Design review of the part built by this model. Coordinates are the model's own, in mm. Face numbers are marked on the shaded views. A direction names the side the tool comes from. Give positions to 0.01 mm unless a question says otherwise; leave off trailing zeros. Loops run counter-clockwise (first coordinate to the right, second up) from the corner with the lowest first, then second, coordinate; pieces in that order, holes last. Notation, with made-up numbers: (42.5, -5.5) -> (77.5, -5.5) arc R33 cw to (77.5, 29.5) -> close; hole circle Ø11 at (7, 12). An arc over 180 degrees is marked (long way). Use CSV: the item, a comma, the result in double quotes. Start each with the question number.
Item 1: Wall thickness on line 1 along X through (y, z) = (1.9, 0); line 2 along X through (y, z) = (1.5, 0); line 3 along Y through (x, z) = (-3.5, -0.5): over which ranges is each line inside the solid? List them lowest first. Write a range as from..to.
Item 2: We need section C-C (y = 0.85). State the section outline as (x, z) points (3 decimals).
Item 3: We need section B-B (x = 0). State the section outline as (y, z) points (3 decimals), plus the area to 4 significant figures.
Item 4: We need section D-D (x = -1.5). State the section outline as (y, z) points, plus the area to 3 significant figures.
Item 5: The part is to be moulded in two halves that separate along X. For the marked faces 1, 2, 3 and 4, say which applies: +X half, -X half, draft (parallel to the pull), parting line (faces both ways), or undercut.
Item 6: For the marked faces 5 and 6, list the 3-axis set-ups (+Z, -Z, +X, -X, +Y, -Y) from which the entire face can be reached by the end or side of a thin tool; tool diameter is ignored.
Item 7: Clearance check with a flat-ended pin moving along its axis: pin 1 (2 mm diameter, centred on x = 0.5, z = 0, fed in from +Y). State where the tip first meets the part, or that it passes through.
Item 8: We need section A-A (z = 0). State the section outline as (x, y) points (3 decimals).
from build123d import *

# Parameters (mm, degrees)
SKETCH_1_R          = 10
EXTRUDE_1_DEPTH     = 2
SKETCH_2_R          = 5
EXTRUDE_2_DEPTH     = 2
SKETCH_3_R          = 1.75
CUT_EXTRUDE_1_DEPTH = 15.696938457
SKETCH_4_R          = 4
CUT_EXTRUDE_2_DEPTH = 3
SCALE_1_SCALE       = 0.5


with BuildPart() as part:
    # 草图1 → 凸台-拉伸1 (new body)
    with BuildSketch(Plane(origin=(0, 0, 0), x_dir=(1, 0, 0), z_dir=(0, 1, 0))):
        with Locations(Location((0, 0, 0), (0, 0, 270))):
            Circle(SKETCH_1_R)
    extrude(amount=EXTRUDE_1_DEPTH)

    # 草图2 → 凸台-拉伸2 (add)
    with BuildSketch(Plane(origin=(0, 2, 0), x_dir=(1, 0, 0), z_dir=(0, 1, 0))):
        with Locations(Location((0, 0, 0), (0, 0, 270))):
            Circle(SKETCH_2_R)
    extrude(amount=EXTRUDE_2_DEPTH)

    # 草图3 → 切除-拉伸1 (cut, through all)
    with BuildSketch(Plane(origin=(0, 4, 0), x_dir=(1, 0, 0), z_dir=(0, 1, 0))):
        with Locations(Location((0, 0, 0), (0, 0, 270))):
            Circle(SKETCH_3_R)
    extrude(amount=-CUT_EXTRUDE_1_DEPTH, mode=Mode.SUBTRACT)

    # 草图4 → 切除-拉伸2 (cut)
    with BuildSketch(Plane(origin=(0, 4, 0), x_dir=(1, 0, 0), z_dir=(0, 1, 0))):
        with Locations(Location((0, 0, 0), (0, 0, 270))):
            Circle(SKETCH_4_R)
    extrude(amount=-CUT_EXTRUDE_2_DEPTH, mode=Mode.SUBTRACT)


with BuildPart() as part_1:
    # 缩放比例1: scaled about (0, 1.148444863, 0)
    add(part.part.scale(SCALE_1_SCALE).moved(Location((0, 0.574222431, 0))))


solid = part_1.part
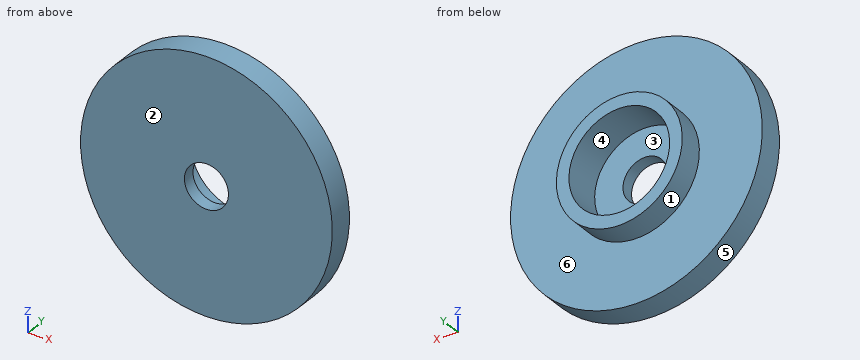
Results found:
1,line 1,"-2.5..-2, 2..2.5"
1,line 2,"-5..-2, 2..5"
1,line 3,"0.57..1.57"
2,outline,"circle Ø10 at (0, 0); hole circle Ø1.75 at (0, 0)"
3,outline,"(0.574, -5) -> (1.574, -5) -> (1.574, -2.5) -> (2.574, -2.5) -> (2.574, -2) -> (1.074, -2) -> (1.074, -0.875) -> (0.574, -0.875) -> close; (0.574, 0.875) -> (1.074, 0.875) -> (1.074, 2) -> (2.574, 2) -> (2.574, 2.5) -> (1.574, 2.5) -> (1.574, 5) -> (0.574, 5) -> close"
3,area,"8.125 mm²"
4,outline,"(0.57, -4.77) -> (1.57, -4.77) -> (1.57, -2) -> (2.57, -2) -> (2.57, -1.32) -> (1.07, -1.32) -> (1.07, 1.32) -> (2.57, 1.32) -> (2.57, 2) -> (1.57, 2) -> (1.57, 4.77) -> (0.57, 4.77) -> close"
4,area,"9.57 mm²"
5,face 1,"parting line"
5,face 2,"draft"
5,face 3,"undercut"
5,face 4,"undercut"
6,face 5,"+Y, -Y"
6,face 6,"+Y"
7,pin 1,"y = 1.07"
8,outline,"(-5, 0.574) -> (-0.875, 0.574) -> (-0.875, 1.074) -> (-2, 1.074) -> (-2, 2.574) -> (-2.5, 2.574) -> (-2.5, 1.574) -> (-5, 1.574) -> close; (0.875, 0.574) -> (5, 0.574) -> (5, 1.574) -> (2.5, 1.574) -> (2.5, 2.574) -> (2, 2.574) -> (2, 1.074) -> (0.875, 1.074) -> close"
